For this review, take the finished solid that the model builds, in its own axes (mm). Face numbers are marked on the shaded views. A direction names the side the tool comes from. Round coordinates to 2 decimals unless told otherwise and drop trailing zeros. Order: outer loops, then holes, each group sorted by start corner. A loop starts at its lowest first (then second) coordinate and runs counter-clockwise, first axis right, second up.
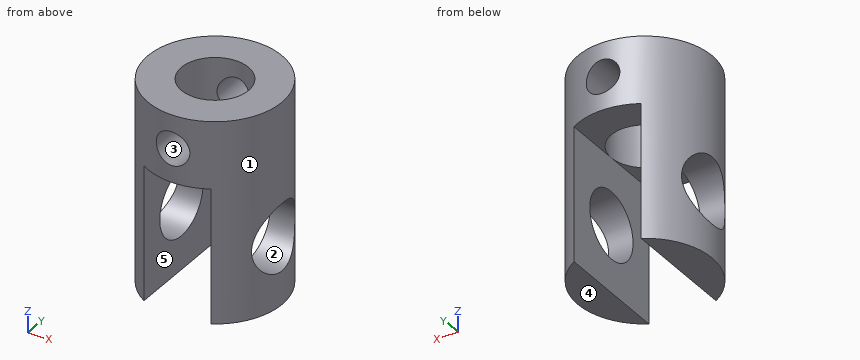
from build123d import *

# Parameters (mm, degrees)
F0_R     = 4
F1_DEPTH = 12
F2_W     = 4
F2_H     = 8
F3_DEPTH = 12.5
F4_R     = 1
F5_DEPTH = 12.5
F6_R     = 2
F7_DEPTH = 12.001
F8_R     = 2
F9_DEPTH = 12.5


with BuildPart() as f1:
    # F0 (on Top) → F1 (new body)
    with BuildSketch(Plane.XY):
        Circle(F0_R)
    extrude(amount=F1_DEPTH)

    # F2 (on Front) → F3 (cut, symmetric)
    with BuildSketch(Plane.XZ):
        with Locations((0, 4)):
            Rectangle(F2_W, F2_H)
    extrude(amount=F3_DEPTH, both=True, mode=Mode.SUBTRACT)

    # F4 (on Front) → F5 (cut, symmetric)
    with BuildSketch(Plane.XZ):
        with Locations((0, 10)):
            Circle(F4_R)
    extrude(amount=F5_DEPTH, both=True, mode=Mode.SUBTRACT)

    # F6 (on face) → F7 (cut, through all)
    with BuildSketch(Plane.XY.offset(12)):
        Circle(F6_R)
    extrude(amount=-F7_DEPTH, mode=Mode.SUBTRACT)

    # F8 (on Right) → F9 (cut, symmetric)
    with BuildSketch(Plane.YZ):
        with Locations((0, 4)):
            Circle(F8_R)
    extrude(amount=F9_DEPTH, both=True, mode=Mode.SUBTRACT)


solid = f1.part
(1) Add section C-C on y = 1.5. Give the boundary of the cut face in (x, z).
(2) Wall thickness on L1, parallel to Z at x = 0, y = -3.5; L2, parallel to Z at x = 3.1, y = 0; L3, parallel to X at y = 2, z = 5.25: over which ranges is each line inside the solid? List them lowest first.
(3) Add section A-A on z = 4. Give the boundary of the cut face in (x, y).
(4) Draft analysis for pull direction Y (two halves, no side actions). For the marked faces 1, 2 and 3, state which applies: pulls with the +Y half, pulls with the -Y half, needs draft (parallel to the pull), parting line crosses it, or undercut.
(5) Clearance check with flat-ended pins moving along their axes: P1, Ø4, axis at x = -1.5, z = 3, coming from the +Y side; P2, Ø1.2, axis at x = 0, y = 1.5, coming from the -Z side; P3, Ø2, axis at x = -3, y = -1, coming from the -Z side; P4, Ø1, axis at y = -1, z = 8, coming from the -X side. State where each tip first meets the part, or that it passes through.
(6) Add section D-D on z = 7.5. Give the boundary of the cut face in (x, y).
(7) Tool access review of the marked faces 4 and 5: name each direction out of +Z, -Z, +X, -X, +Y, -Y from which nothing blocks a thin tool from reaching the whole face with its end or side.
(8) Add section B-B on x = 0. Give the boundary of the cut face in (y, z).
Here are the results:
1. outline: (-3.71, 0) - (-2, 0) - (-2, 2.68) - (-3.71, 2.68) - close; (-3.71, 5.32) - (-2, 5.32) - (-2, 8) - (-1.32, 8) - (-1.32, 12) - (-3.71, 12) - close; (1.32, 8) - (2, 8) - (2, 5.32) - (3.71, 5.32) - (3.71, 12) - (1.32, 12) - close; (2, 0) - (3.71, 0) - (3.71, 2.68) - (2, 2.68) - close
2. L1: z = 8 to 9, 11 to 12
2. L2: z = 0 to 2, 6 to 12
2. L3: x = -3.46 to -2, 2 to 3.46
3. outline: (-3.46, -2) arc R4 ccw to (-2, -3.46) - (-2, -2) - close; (-3.46, 2) - (-2, 2) - (-2, 3.46) arc R4 ccw to start; (2, -3.46) arc R4 ccw to (3.46, -2) - (2, -2) - close; (2, 2) - (3.46, 2) arc R4 ccw to (2, 3.46) - close
4. face 1: parting line crosses it
4. face 2: undercut
4. face 3: needs draft
5. P1: stops at y = 3.46
5. P2: stops at z = 8
5. P3: stops at z = 0
5. P4: stops at x = -3.97
6. outline: (-2, -3.46) - (-2, 3.46) arc R4 ccw to start; (2, -3.46) arc R4 ccw to (2, 3.46) - close
7. face 4: -Z, +X, -X, +Y, -Y
7. face 5: -Z, +Y, -Y
8. outline: (-4, 8) - (-2, 8) - (-2, 9) - (-4, 9) - close; (-4, 11) - (-2, 11) - (-2, 12) - (-4, 12) - close; (2, 8) - (4, 8) - (4, 9) - (2, 9) - close; (2, 11) - (4, 11) - (4, 12) - (2, 12) - close
